Verification items for the finished model (mm, model axes). Face numbers are marked on the shaded views. A direction names the side the tool comes from. Round coordinates to 2 decimals unless told otherwise and drop trailing zeros. Write each loop counter-clockwise with the first axis right and the second up, starting at its lowest first coordinate (ties: lowest second). Pieces come first, ordered by that corner, then holes. Notation, with made-up numbers: M 87.5,46 L 126.5,46 A5 ccw 126.5,55 Z; hole C 33,6 d10. An arc over 180 degrees is marked long. One line per question, with ' | ' between items.
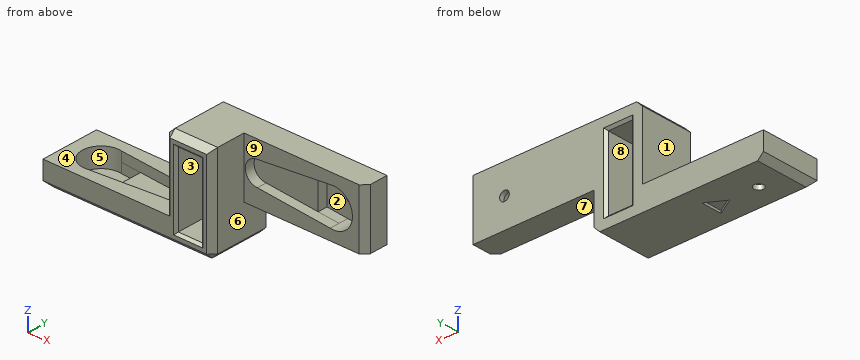
from build123d import *

# Parameters (mm, degrees)
SKETCH1_W               = 35
SKETCH1_H               = 12.2
BOSS_EXTRUDE1_DEPTH     = 5
SKETCH2_R               = 1
CUT_EXTRUDE1_DEPTH      = 38.775970389
SKETCH3_W               = 10
SKETCH3_H               = 12.2
BOSS_EXTRUDE2_DEPTH     = 15
SKETCH4_W               = 12.2
SKETCH4_H               = 5
BOSS_EXTRUDE3_DEPTH     = 25
CUT_EXTRUDE2_DEPTH      = 42.419255471
CUT_EXTRUDE2_DEPTH_BACK = 42.419255471
SKETCH5_R               = 1
CUT_EXTRUDE3_DEPTH      = 0.5
CHAMFER1_SIZE           = 1.2
SKETCH8_R               = 3.9
CUT_EXTRUDE4_DEPTH      = 4
CUT_EXTRUDE5_DEPTH      = 2
CUT_EXTRUDE6_DEPTH      = 4
SKETCH20_R              = 3.9
CUT_EXTRUDE11_DEPTH     = 4
CUT_EXTRUDE12_DEPTH     = 2
CUT_EXTRUDE13_DEPTH     = 4
SKETCH23_W              = 5
SKETCH23_H              = 15
CUT_EXTRUDE14_DEPTH     = 43.574108608
CHAMFER2_SIZE           = 0.5


with BuildPart() as part:
    # Sketch1 → Boss-Extrude1 (new body)
    with BuildSketch(Plane.XY):
        with Locations((-18.048765432, 5.660493827)):
            Rectangle(SKETCH1_W, SKETCH1_H)
    extrude(amount=BOSS_EXTRUDE1_DEPTH)

    # Sketch2 → Cut-Extrude1 (cut, through all)
    with BuildSketch(Plane.XY.offset(5)):
        with Locations((-29.048765432, 5.660493827)):
            Circle(SKETCH2_R)
    extrude(amount=-CUT_EXTRUDE1_DEPTH, mode=Mode.SUBTRACT)

    # Sketch3 → Boss-Extrude2 (add)
    with BuildSketch(Plane.XY.offset(5)):
        with Locations((-5.548765432, 5.660493827)):
            Rectangle(SKETCH3_W, SKETCH3_H)
    extrude(amount=BOSS_EXTRUDE2_DEPTH)

    # Sketch4 → Boss-Extrude3 (add)
    with BuildSketch(Plane(origin=(-0.548765432, 0, 0), x_dir=(0, 0, -1), z_dir=(1, 0, 0))):
        with Locations((-13.9, 9.260493827)):
            Rectangle(SKETCH4_W, SKETCH4_H)
    extrude(amount=BOSS_EXTRUDE3_DEPTH)

    # Sketch5 → Cut-Extrude2 (cut, two sides: drawn at the far end of the back side and taken through both)
    with BuildSketch(Plane.XZ.offset(-6.760493827).offset(-CUT_EXTRUDE2_DEPTH_BACK)):
        with Locations(Location((17.951234568, 13.9, 0), (0, 0, 270))):
            Circle(SKETCH5_R)
    extrude(amount=CUT_EXTRUDE2_DEPTH + CUT_EXTRUDE2_DEPTH_BACK, mode=Mode.SUBTRACT)

    # Sketch7 → Cut-Extrude3 (cut)
    with BuildSketch(Plane(origin=(0, 0, 0), x_dir=(-1, 0, 0), z_dir=(0, 0, -1))):
        Polygon((23.048765432, 5.660493827), (19.298765432, 7.825557337), (19.298765432, 3.495430318), align=None)
    extrude(amount=-CUT_EXTRUDE3_DEPTH, mode=Mode.SUBTRACT)

    # Chamfer1
    chamfer1_edges = [part.edges().sort_by_distance(p)[0] for p in [
        (-10.548765432, -0.439506173, 12.5),
        (-10.548765432, 5.660493827, 20),
        (-5.548765432, -0.439506173, 20),
        (24.451234568, 6.760493827, 13.9),
        (-0.548765432, 5.660493827, 0),
        (-18.048765432, -0.439506173, 0),
        (-35.548765432, 5.660493827, 0),
        (-0.548765432, -0.439506173, 10),
    ]]
    chamfer(chamfer1_edges, length=CHAMFER1_SIZE)

    # Sketch8 → Cut-Extrude4 (cut)
    with BuildSketch(Plane.XY.offset(5)):
        with Locations((-29.048765432, 5.660493827)):
            Circle(SKETCH8_R)
    extrude(amount=-CUT_EXTRUDE4_DEPTH, mode=Mode.SUBTRACT)

    # Sketch10 → Cut-Extrude5 (cut)
    with BuildSketch(Plane.XY.offset(5)):
        with BuildLine():
            Line((-29.048765432, 9.560493827), (-13.548765432, 8.160493827))
            ThreePointArc((-13.548765432, 8.160493827), (-11.048765432, 5.660493827), (-13.548765432, 3.160493827))
            Line((-13.548765432, 3.160493827), (-29.048765432, 1.760493827))
            Line((-29.048765432, 1.760493827), (-29.048765432, 9.560493827))
        make_face()
    extrude(amount=-CUT_EXTRUDE5_DEPTH, mode=Mode.SUBTRACT)

    # Sketch12 → Cut-Extrude6 (cut)
    with BuildSketch(Plane.XY.offset(5)):
        Polygon((-24.048765432, 5.660493827), (-24.048765432, 9.108880924), (-29.048765432, 9.560493827), (-29.048765432, 1.760493827), (-24.048765432, 2.21210673), align=None)
    extrude(amount=-CUT_EXTRUDE6_DEPTH, mode=Mode.SUBTRACT)

    # Sketch20 → Cut-Extrude11 (cut)
    with BuildSketch(Plane.XZ.offset(-6.760493827)):
        with Locations(Location((17.951234568, 13.9, 0), (0, 0, 270))):
            Circle(SKETCH20_R)
    extrude(amount=-CUT_EXTRUDE11_DEPTH, mode=Mode.SUBTRACT)

    # Sketch21 → Cut-Extrude12 (cut)
    with BuildSketch(Plane.XZ.offset(-6.760493827)):
        with BuildLine():
            Line((17.951234568, 17.8), (2.21295028, 16.4))
            ThreePointArc((2.21295028, 16.4), (-0.28704972, 13.9), (2.21295028, 11.4))
            Line((2.21295028, 11.4), (17.951234568, 10))
            Line((17.951234568, 10), (17.951234568, 17.8))
        make_face()
    extrude(amount=-CUT_EXTRUDE12_DEPTH, mode=Mode.SUBTRACT)

    # Sketch22 → Cut-Extrude13 (cut)
    with BuildSketch(Plane.XZ.offset(-6.760493827)):
        Polygon((17.951234568, 17.8), (17.951234568, 10), (12.951234568, 10.444775293), (12.951234568, 17.355224707), align=None)
    extrude(amount=-CUT_EXTRUDE13_DEPTH, mode=Mode.SUBTRACT)

    # Sketch23 → Cut-Extrude14 (cut, through all)
    with BuildSketch(Plane(origin=(0, 11.760493827, 0), x_dir=(1, 0, 0), z_dir=(0, 1, 0))):
        with Locations((-5.548765432, -10)):
            Rectangle(SKETCH23_W, SKETCH23_H)
    extrude(amount=-CUT_EXTRUDE14_DEPTH, mode=Mode.SUBTRACT)

    # Chamfer2
    chamfer2_edges = [part.edges().sort_by_distance(p)[0] for p in [
        (-8.048765432, -0.439506173, 10),
        (-5.548765432, -0.439506173, 2.5),
        (-3.048765432, -0.439506173, 10),
        (-5.548765432, -0.439506173, 17.5),
        (-8.048765432, 11.760493827, 10),
        (-5.548765432, 11.760493827, 17.5),
        (-3.048765432, 11.760493827, 10),
        (-5.548765432, 11.760493827, 2.5),
    ]]
    chamfer(chamfer2_edges, length=CHAMFER2_SIZE)


solid = part.part
1. Thickness scan on line 1 (X direction, y = 8.25, z = 14); line 2 (X direction, y = 11.25, z = 13.9); line 3 (X direction, y = 3.25, z = 13). Record the ranges inside material, lowest first.
Results:
line 1: x = -10.55 to -8.05, -3.05 to -0.29, 21.85 to 24.45 | line 2: x = -10.55 to -8.05, -3.05 to 16.95, 18.95 to 24.45 | line 3: x = -10.55 to -8.05, -3.05 to -0.55
2. Tool access check on the marked faces 5, 6, 7, 8 and 9. Record the directions out of +Z, -Z, +X, -X, +Y, -Y that give a thin tool (end or side, any length) a straight path to the whole face; none if there is none.
Results:
face 5: +Z | face 6: -Z, +X, -Y | face 7: -Z, +X, +Y, -Y | face 8: +Y, -Y | face 9: +Z, -Z, +X, -Y
3. Section check C-C, the plane x = -20.5. Record the cut outline in (y, z), then the cut area to 3 significant figures.
Results:
outline: M -0.44,1.2 L 0.76,0 L 4.19,0 L 4.19,0.5 L 7.13,0.5 L 7.13,0 L 11.76,0 L 11.76,5 L 8.79,5 L 8.79,3 L 2.53,3 L 2.53,5 L -0.44,5 Z | area: 46.3 mm2
4. Mould release check, pull along Z, two halves, no side actions. Record for the marked faces 1, 2, 3 and 4: pulls with the +Z half, pulls with the -Z half, needs draft (parallel to the pull), parting line crosses it, or undercut.
Results:
face 1: needs draft | face 2: undercut | face 3: undercut | face 4: pulls with the +Z half
5. Section check A-A, the plane z = 13.9. Record the cut outline in (x, y), then the cut area to 3 significant figures.
Results:
outline: M -10.55,0.76 L -9.35,-0.44 L -8.55,-0.44 L -8.05,0.06 L -8.05,11.26 L -8.55,11.76 L -10.55,11.76 Z; M -3.05,0.06 L -2.55,-0.44 L -1.75,-0.44 L -0.55,0.76 L -0.55,6.76 L -0.29,6.76 L -0.29,8.76 L 12.95,8.76 L 12.95,10.76 L 16.95,10.76 L 16.95,11.76 L -2.55,11.76 L -3.05,11.26 Z; M 18.95,10.76 L 21.85,10.76 L 21.85,6.76 L 23.25,6.76 L 24.45,7.96 L 24.45,11.76 L 18.95,11.76 Z | area: 119 mm2
6. Section check B-B, the plane x = 6.5. Record the cut outline in (y, z).
Results:
outline: M 6.76,7.8 L 11.76,7.8 L 11.76,20 L 6.76,20 L 6.76,16.78 L 8.76,16.78 L 8.76,11.02 L 6.76,11.02 Z
7. Go/stop test with flat-tipped pins: P1, Ø5.5, axis at x = 4.5, z = 13, coming from the -Y side; P2, Ø1.6, axis at x = -29.05, y = 5.66, coming from the +Z side; P3, Ø5.5, axis at x = -19, y = 4.5, coming from the +Z side; P4, Ø3, axis at y = 2, z = 8.5, coming from the +X side. Record where each tip stops, or that it passes through.
Results:
P1: stops at y = 6.76 | P2: passes through | P3: stops at z = 5 | P4: stops at x = -0.55
